Can you work these out from the drawing? Everything is in mm from the part's minimum corner. A direction names the side the tool comes from. Coordinates: 2 decimals unless noted, no trailing zeros. Loops run counter-clockwise (first coordinate to the right, second up) from the corner with the lowest first, then second, coordinate; pieces in that order, holes last. Notation, with made-up numbers: (23.5, -17.75) -> (74.5, -17.75) arc R20 cw to (74.5, 2.25) -> close; hole circle Ø4 at (40, -0.5). An arc over 180 degrees is marked (long way). Put each result on its own line as item: value. Start each with the question number.
Item 1: For the marked faces 4, 5, 6 and 7, which set-ups out of +Z, -Z, +X, -X, +Y, -Y let a thin tool reach every point of the face, with its end or its side?
Item 2: If we section it at A-A on z = 38.1: Please give me the cut outline in (x, y).
Item 3: If we section it at C-C on y = 32: Please give me the cut outline in (x, z).
Item 4: If we section it at B-B on x = 63.5: Please give me the cut outline in (y, z), plus the area to 3 significant figures.
Item 5: We'd pull the mould along X, two halves only. Please class the marked faces 1, 2 and 3: pulls with the +X half, pulls with the -X half, needs draft (parallel to the pull), parting line crosses it, or undercut.
Item 6: Please list where these lines run through material, in increasing order: L1, parallel to X at y = 15.25, z = 38.1; L2, parallel to Z at x = 63, y = 32; L3, parallel to Z at x = 63.5, y = 9.25. Write a range as from..to.
Item 7: Will these pins go through, and if not, where does the flat tip stop? P1, Ø5.5, axis at x = 43.5, y = 31, coming from the -Z side; P2, Ø1.5, axis at x = 69, z = 56, coming from the +Y side; P3, Ø5, axis at y = 3.5, z = 33.5, coming from the -X side; P4, Ø5, axis at x = 116.5, z = 39, coming from the -Y side.
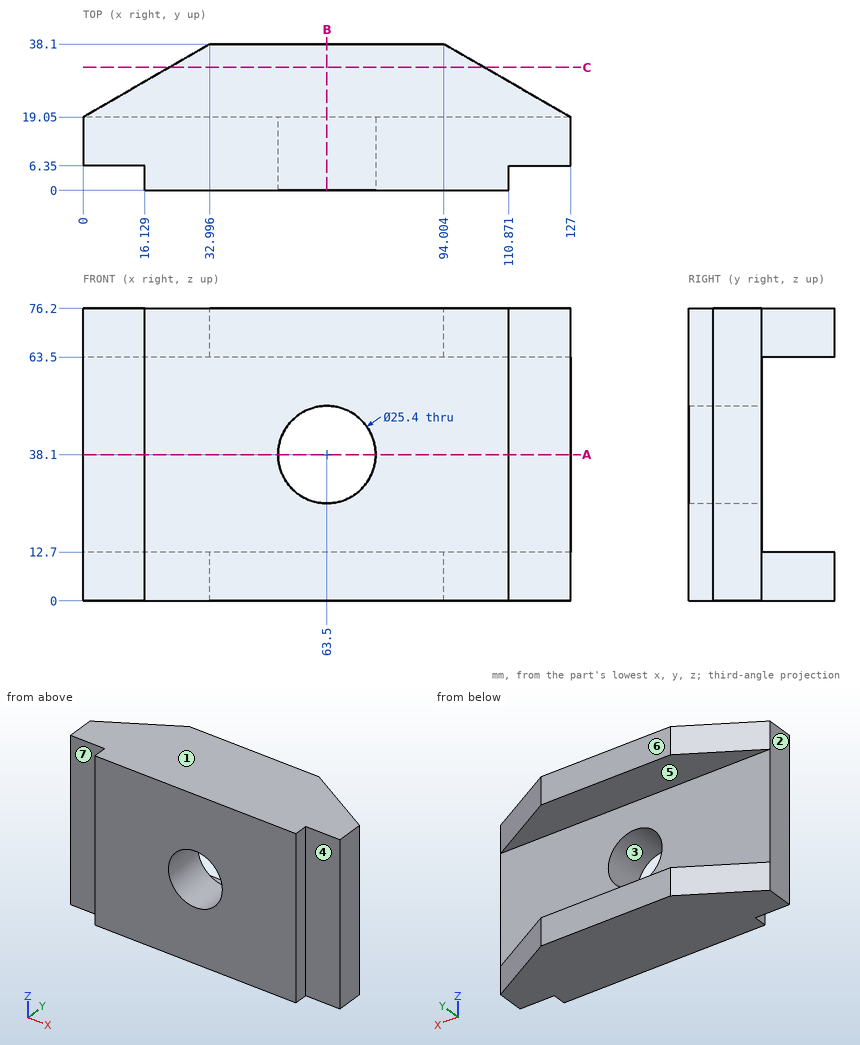
Solutions:
1. face 4: +Z, -Z, +X, -Y
1. face 5: +X, -X, +Y
1. face 6: +Z, -Z, +X, -X, +Y
1. face 7: +Z, -Z, -X, -Y
2. outline: (0, 6.35) -> (16.13, 6.35) -> (16.13, 0) -> (50.8, 0) -> (50.8, 19.05) -> (0, 19.05) -> close; (76.2, 0) -> (110.87, 0) -> (110.87, 6.35) -> (127, 6.35) -> (127, 19.05) -> (76.2, 19.05) -> close
3. outline: (22.43, 0) -> (104.57, 0) -> (104.57, 12.7) -> (22.43, 12.7) -> close; (22.43, 63.5) -> (104.57, 63.5) -> (104.57, 76.2) -> (22.43, 76.2) -> close
4. outline: (0, 0) -> (38.1, 0) -> (38.1, 12.7) -> (19.05, 12.7) -> (19.05, 25.4) -> (0, 25.4) -> close; (0, 50.8) -> (19.05, 50.8) -> (19.05, 63.5) -> (38.1, 63.5) -> (38.1, 76.2) -> (0, 76.2) -> close
4. area: 1,450 mm^2
5. face 1: needs draft
5. face 2: pulls with the -X half
5. face 3: undercut
6. L1: 0..50.8, 76.2..127
6. L2: 0..12.7, 63.5..76.2
6. L3: 0..25.4, 50.8..76.2
7. P1: z = 0
7. P2: y = 19.05
7. P3: x = 16.13
7. P4: y = 6.35
